from build123d import *

# Parameters (mm, degrees)
F0_R     = 56.020962
F1_DEPTH = 68.58
F4_DEPTH = 67.818
F5_R     = 5.08


with BuildPart() as f1:
    # F0 (on Top) → F1 (new body)
    with BuildSketch(Plane.XY):
        Circle(F0_R)
    extrude(amount=F1_DEPTH)

    # F3 (on offset) → F4 (cut)
    with BuildSketch(Plane.YZ.offset(33.782)):
        with BuildLine():
            ThreePointArc((0, 43.215101), (18.128478, 50.724162), (25.63754, 68.852641))
            ThreePointArc((25.63754, 68.852641), (-18.128478, 86.981119), (0, 43.215101))
        make_face()
    extrude(amount=-F4_DEPTH, mode=Mode.SUBTRACT)

    # F5
    f5_edges = [f1.edges().sort_by_distance(p)[0] for p in [
        (-56.020962, 0, 68.58),
    ]]
    fillet(f5_edges, radius=F5_R)


solid = f1.part
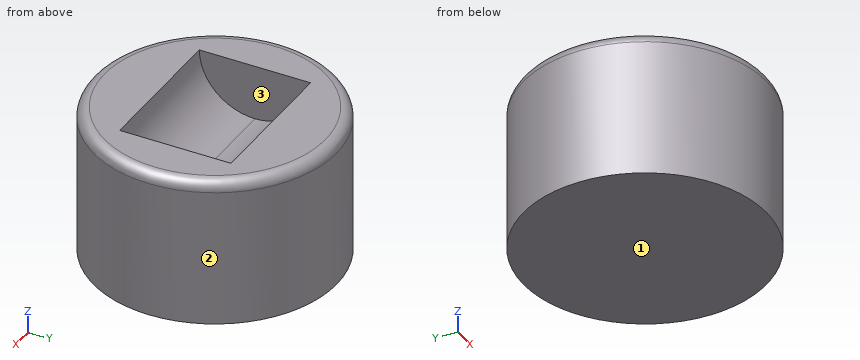
Verification items for the finished model (mm, model axes). Face numbers are marked on the shaded views. Round coordinates to 2 decimals unless told otherwise and drop trailing zeros. Loops run counter-clockwise (first coordinate to the right, second up) from the corner with the lowest first, then second, coordinate; pieces in that order, holes last. Notation, with made-up numbers: (2, -36.75) - (54, -36.75) arc R24 ccw to (54, -16.75) - close; hole circle Ø6 at (-30, 3.5). An arc over 180 degrees is marked (long way). Answer in a Markdown table with one row per item. Add a question column.
Q1. Section check A-A on x = 0. Enter the section's corners in (y, z), plus the area to 3 significant figures.
Q2. Material ranges on line 1 (X direction, y = -2, z = 49); line 2 (X direction, y = -19, z = 62); line 3 (Y direction, x = 4, z = 66.5), recorded low to high.
Q3. Gauge pin test, flat ends, axial feed: pin 1 (1.5 mm diameter, centred on y = 35.5, z = 58, fed in from -X); pin 2 (10 mm diameter, centred on y = -22, z = 10.5, fed in from +X); pin 3 (10 mm diameter, centred on x = 29.5, z = 59.5, fed in from -Y). Record the tip position at first contact, or that the pin passes through.
Q4. Release check for a two-part mould opening along Y. For the marked faces 1, 2 and 3 record: pulls with the +Y half, pulls with the -Y half, needs draft (parallel to the pull), parting line crosses it, or undercut.
Q5. Section check B-B on z = 11.5. Enter the section's corners in (x, y), plus the area to 3 significant figures.
Q6. Section check C-C on z = 56.5. Enter the section's corners in (x, y), plus the area to 3 significant figures.
Found:
| question | item | result |
|---|---|---|
| 1 | outline | (-56.02, 0) - (56.02, 0) - (56.02, 63.5) arc R5.08 ccw to (50.94, 68.58) - (25.64, 68.58) arc R25.64 cw to (-25.64, 68.58) - (-50.94, 68.58) arc R5.08 ccw to (-56.02, 63.5) - close |
| 1 | area | 6,650 mm² |
| 2 | line 1 | x = -55.99 to -34.04, 33.78 to 55.99 |
| 2 | line 2 | x = -52.7 to -34.04, 33.78 to 52.7 |
| 2 | line 3 | y = -54.89 to -25.53, 25.53 to 54.89 |
| 3 | pin 1 | stops at x = -43.94 |
| 3 | pin 2 | stops at x = 53.38 |
| 3 | pin 3 | stops at y = -50.38 |
| 4 | face 1 | needs draft |
| 4 | face 2 | parting line crosses it |
| 4 | face 3 | undercut |
| 5 | outline | circle Ø112.04 at (0, 0) |
| 5 | area | 9,860 mm² |
| 6 | outline | circle Ø112.04 at (0, 0); hole (-34.04, -22.47) - (33.78, -22.47) - (33.78, 22.47) - (-34.04, 22.47) - close |
| 6 | area | 6,810 mm² |
